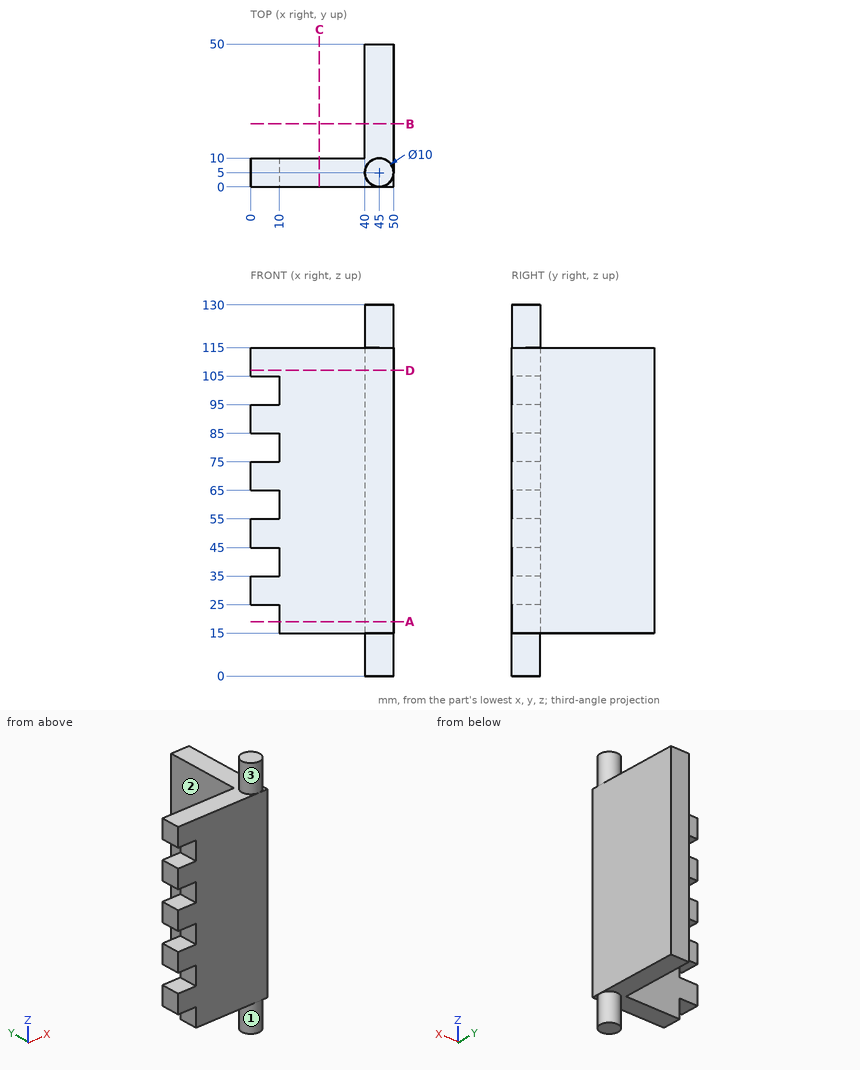
Here's the drawing with two shaded views (mm, measured from the low corner). I have some questions. A direction names the side the tool comes from. Give positions to 0.01 mm unless a question says otherwise; leave off trailing zeros. Loops run counter-clockwise (first coordinate to the right, second up) from the corner with the lowest first, then second, coordinate; pieces in that order, holes last. Notation, with made-up numbers: M 19,14 L 52,14 A18 cw 52,26 Z; hole C 19.5,63 d8. An arc over 180 degrees is marked long. One line per item, written item: value. Start each with the question number.
1) If I drill on line 1 (Z direction, x = 8.5, y = 9.5); line 2 (Z direction, x = 41.5, y = 38); line 3 (X direction, y = 8.5, z = 20), over which ranges is the centre line in solid material (lowest first)? Write a range as [from, to].
2) If we section it at D-D, the plane z = 107: Write out the boundary of the cut face in (x, y).
3) If we section it at C-C, the plane x = 24: Write out the boundary of the cut face in (y, z).
4) I'm going to push flat-ended pins straight in: pin 1 (1 mm diameter, centred on y = 34, z = 94.5, fed in from -X); pin 2 (5 mm diameter, centred on x = 3.5, y = 3.5, fed in from -Z); pin 3 (11 mm diameter, centred on x = 3.5, y = 4.5, fed in from +Z). Where does each tip first touch, or does it pass through?
5) If we section it at A-A, the plane z = 19: Write out the boundary of the cut face in (x, y), and give its area (3 significant figures).
6) On a 3-axis mill with a long thin cutter (end or side, diameter ignored), from which of +Z, -Z, +X, -X, +Y, -Y can I reach the whole of each face in a straight line? I mean the marked faces 1, 2 and 3. Say none if no direction works.
7) If we section it at B-B, the plane y = 22: Write out the boundary of the cut face in (x, z).
Completed:
1. line 1: z = [25, 35], [45, 55], [65, 75], [85, 95], [105, 115]
1. line 2: z = [15, 115]
1. line 3: x = [10, 50]
2. outline: M 0,0 L 50,0 L 50,50 L 40,50 L 40,10 L 0,10 Z
3. outline: M 0,15 L 10,15 L 10,115 L 0,115 Z
4. pin 1: stops at x = 40
4. pin 2: stops at z = 25
4. pin 3: stops at z = 115
5. outline: M 10,0 L 50,0 L 50,50 L 40,50 L 40,10 L 10,10 Z
5. area: 800 mm^2
6. face 1: -Z
6. face 2: +Z, -Z, -X, +Y
6. face 3: +Z
7. outline: M 40,15 L 50,15 L 50,115 L 40,115 Z
